```python
from build123d import *

# Parameters (mm, degrees)
SKETCH1_R               = 11
BOSS_EXTRUDE1_DEPTH     = 40
BOSS_EXTRUDE2_DEPTH     = 32
SKETCH4_W               = 144
SKETCH4_H               = 40
BOSS_EXTRUDE4_DEPTH     = 5
BOSS_EXTRUDE5_DEPTH     = 32
CUT_EXTRUDE2_DEPTH      = 3
SKETCH6_W               = 120
SKETCH6_H               = 20
CUT_EXTRUDE3_DEPTH      = 5
SKETCH8_W               = 2
SKETCH8_H               = 40
CUT_EXTRUDE_THIN1_DEPTH = 18
FILLET2_R               = 5
SKETCH9_R               = 2.25
CUT_EXTRUDE4_DEPTH      = 226
CUT_EXTRUDE5_START      = -3
CUT_EXTRUDE5_DEPTH      = 11
BOSS_EXTRUDE6_DEPTH     = 40
FILLET3_R               = 2


with BuildPart() as part:
    # Sketch1 → Boss-Extrude1 (new body)
    with BuildSketch(Plane(origin=(0, 0, 0), x_dir=(1, 0, 0), z_dir=(0, 1, 0))):
        with BuildLine():
            Line((137.460581558, -14.5), (119.460581558, -14.5))
            Line((119.460581558, -14.5), (119.460581558, 7.5))
            Line((119.460581558, 7.5), (-24.539418442, 7.5))
            Line((-24.539418442, 7.5), (-24.539418442, -14.5))
            Line((-24.539418442, -14.5), (-42.539418442, -14.5))
            Line((-42.539418442, -14.5), (-56.539418442, -14.5))
            Line((-56.539418442, -14.5), (-56.539418442, -0.5))
            ThreePointArc((-56.539418442, -0.5), (-52.438913379, 9.399494937), (-42.539418442, 13.5))
            Line((-42.539418442, 13.5), (137.460581558, 13.5))
            ThreePointArc((137.460581558, 13.5), (147.360076494, 9.399494937), (151.460581558, -0.5))
            Line((151.460581558, -0.5), (151.460581558, -14.5))
            Line((151.460581558, -14.5), (137.460581558, -14.5))
        make_face()
        with Locations((-42.539418442, -0.5)):
            Circle(SKETCH1_R, mode=Mode.SUBTRACT)
        with Locations((137.460581558, -0.5)):
            Circle(SKETCH1_R, mode=Mode.SUBTRACT)
    extrude(amount=BOSS_EXTRUDE1_DEPTH)

    # Sketch2 → Boss-Extrude2 (add)
    with BuildSketch(Plane.ZY.offset(56.539418442)):
        with BuildLine():
            Line((14.5, 40), (19, 40))
            ThreePointArc((19, 40), (22.535533906, 38.535533906), (24, 35))
            Line((24, 35), (24, 29))
            ThreePointArc((24, 29), (15, 20), (24, 11))
            Line((24, 11), (24, 5))
            ThreePointArc((24, 5), (22.535533906, 1.464466094), (19, 0))
            Line((19, 0), (14.5, 0))
            Line((14.5, 0), (14.5, 40))
        make_face()
    extrude(amount=-BOSS_EXTRUDE2_DEPTH)

    # Sketch4 → Boss-Extrude4 (add)
    with BuildSketch(Plane.XY.offset(-7.5)):
        with Locations((47.460581558, 20)):
            Rectangle(SKETCH4_W, SKETCH4_H)
    extrude(amount=BOSS_EXTRUDE4_DEPTH)

    # Sketch3 → Boss-Extrude5 (add)
    with BuildSketch(Plane(origin=(151.460581558, 0, 0), x_dir=(0, 0, -1), z_dir=(1, 0, 0))):
        with BuildLine():
            Line((-24, 11), (-24, 5))
            ThreePointArc((-24, 5), (-22.535533906, 1.464466094), (-19, 0))
            Line((-19, 0), (-14.5, 0))
            Line((-14.5, 0), (-14.5, 40))
            Line((-14.5, 40), (-19, 40))
            ThreePointArc((-19, 40), (-22.535533906, 38.535533906), (-24, 35))
            Line((-24, 35), (-24, 29))
            ThreePointArc((-24, 29), (-15, 20), (-24, 11))
        make_face()
    extrude(amount=-BOSS_EXTRUDE5_DEPTH)

    # Sketch5 → Cut-Extrude2 (cut)
    with BuildSketch(Plane(origin=(0, 0, -13.5), x_dir=(-1, 0, 0), z_dir=(0, 0, -1))):
        with BuildLine():
            Line((32.539418442, 35), (-127.460581558, 35))
            ThreePointArc((-127.460581558, 35), (-130.996115464, 33.535533906), (-132.460581558, 30))
            Line((-132.460581558, 30), (-132.460581558, 10))
            ThreePointArc((-132.460581558, 10), (-130.996115464, 6.464466094), (-127.460581558, 5))
            Line((-127.460581558, 5), (32.539418442, 5))
            ThreePointArc((32.539418442, 5), (36.074952348, 6.464466094), (37.539418442, 10))
            Line((37.539418442, 10), (37.539418442, 30))
            ThreePointArc((37.539418442, 30), (36.074952348, 33.535533906), (32.539418442, 35))
        make_face()
    extrude(amount=-CUT_EXTRUDE2_DEPTH, mode=Mode.SUBTRACT)

    # Sketch6 → Cut-Extrude3 (cut)
    with BuildSketch(Plane(origin=(0, 0, -10.5), x_dir=(-1, 0, 0), z_dir=(0, 0, -1))):
        with Locations((-47.460581558, 20)):
            Rectangle(SKETCH6_W, SKETCH6_H)
    extrude(amount=-CUT_EXTRUDE3_DEPTH, mode=Mode.SUBTRACT)

    # Sketch8 → Cut-Extrude-Thin1 (cut)
    with BuildSketch(Plane(origin=(0, 0, -13.5), x_dir=(-1, 0, 0), z_dir=(0, 0, -1))):
        with Locations((-137.460581558, 20)):
            Rectangle(SKETCH8_W, SKETCH8_H)
        with Locations((42.539418442, 20)):
            Rectangle(SKETCH8_W, SKETCH8_H)
    extrude(amount=-CUT_EXTRUDE_THIN1_DEPTH, mode=Mode.SUBTRACT)

    # Fillet2
    fillet2_edges = [part.edges().sort_by_distance(p)[0] for p in [
        (138.460581558, 0, -11.959345597),
        (138.460581558, 40, -11.959345597),
        (136.460581558, 0, -11.977225575),
        (136.460581558, 40, -11.977225575),
        (-41.539418442, 40, -11.977225575),
        (-43.539418442, 40, -11.959345597),
        (-43.539418442, 0, -11.959345597),
        (-41.539418442, 0, -11.977225575),
    ]]
    fillet(fillet2_edges, radius=FILLET2_R)

    # Sketch9 → Cut-Extrude4 (cut)
    with BuildSketch(Plane(origin=(151.460581558, 0, 0), x_dir=(0, 0, -1), z_dir=(1, 0, 0))):
        with Locations((-0.5, 20)):
            Circle(SKETCH9_R)
    extrude(amount=-CUT_EXTRUDE4_DEPTH, mode=Mode.SUBTRACT)

    # Sketch10 → Cut-Extrude5 (cut)
    with BuildSketch(Plane(origin=(-24.539418442, 0, 0), x_dir=(0, 0, -1), z_dir=(1, 0, 0)).offset(CUT_EXTRUDE5_START)):
        Polygon((-0.5, 24.156921938), (-4.1, 22.078460969), (-4.1, 17.921539031), (-0.5, 15.843078062), (3.1, 17.921539031), (3.1, 22.078460969), align=None)
    cut_extrude5 = extrude(amount=CUT_EXTRUDE5_DEPTH, mode=Mode.SUBTRACT)

    # Mirror5: Cut-Extrude5 across plane
    add(cut_extrude5.mirror(Plane.ZY.offset(-47.460581558)), mode=Mode.SUBTRACT)

    # Sketch12 → Boss-Extrude6 (add)
    with BuildSketch(Plane(origin=(0, 0, 0), x_dir=(-1, 0, 0), z_dir=(0, -1, 0))):
        with BuildLine():
            Line((-103.460581558, -3.5), (-103.460581558, 2.5))
            Line((-103.460581558, 2.5), (-100.460581558, 2.5))
            Line((-100.460581558, 2.5), (-100.460581558, -3.5))
            ThreePointArc((-100.460581558, -3.5), (-103.243067136, -10.217514421), (-109.960581558, -13))
            Line((-109.960581558, -13), (-119.460581558, -13))
            Line((-119.460581558, -13), (-119.460581558, -10))
            Line((-119.460581558, -10), (-116.460581558, -10))
            Line((-116.460581558, -10), (-109.960581558, -10))
            ThreePointArc((-109.960581558, -10), (-105.36438748, -8.096194078), (-103.460581558, -3.5))
        make_face()
    extrude(amount=-BOSS_EXTRUDE6_DEPTH)

    # Fillet3
    fillet3_edges = [part.edges().sort_by_distance(p)[0] for p in [
        (119.460581558, 20, 10),
    ]]
    fillet(fillet3_edges, radius=FILLET3_R)


solid = part.part
```
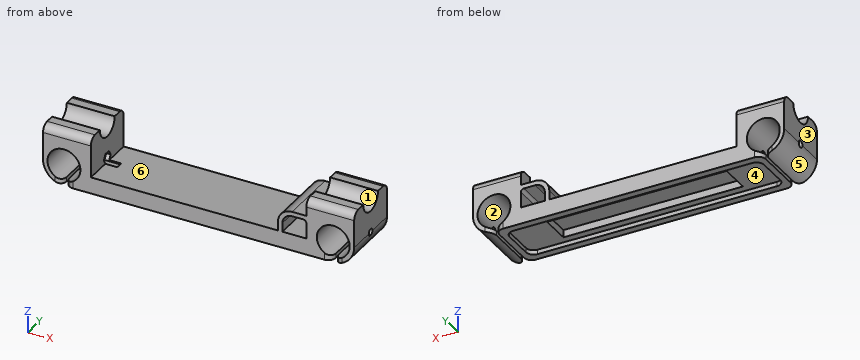
CAD build for the part. Positions are in the model's coordinates, mm. Face numbers are marked on the shaded views. A direction names the side the tool comes from. Round coordinates to 2 decimals unless told otherwise and drop trailing zeros. Loops run counter-clockwise (first coordinate to the right, second up) from the corner with the lowest first, then second, coordinate; pieces in that order, holes last. Notation, with made-up numbers: M 38,-32 L 60,-32 A18 ccw 60,-11 Z; hole C 28.5,81 d3. An arc over 180 degrees is marked long. Return JSON: item names as keys, results as strings. Group by question number.
(1) Drop flat-ended pins along their axis: P1, Ø15, axis at x = 60.5, y = 24, coming from the -Z side; P2, Ø3.5, axis at y = 20, z = 0.5, coming from the +X side; P3, Ø2.5, axis at y = 19.5, z = -11.5, coming from the -X side. Give the stop position or say it passes through.
(2) Saw through at D-D, the plane x = -21. List the corners of the cut face in (y, z), and give its area (3 significant figures).
(3) Tool access for the marked faces 4, 5 and 6: list every direction of +Z, -Z, +X, -X, +Y, -Y with a clear straight run to the whole face (end or side of a thin tool).
(4) Saw through at A-A, the plane x = 88.5. List the corners of the cut face in (y, z).
(5) Wall check: probe 1 along X at (y, z) = (29, 0); probe 2 along X at (y, z) = (5.5, -3); probe 3 along X at (y, z) = (7, 15.5). Give the ranges that are in metal, low to high. Write a range as [from, to].
(6) Mould opens along X. For the marked faces 1, 2 and 3 say: +X half, -X half, draft (parallel to the pull), parting line (faces both ways), or undercut.
(7) Saw through at B-B, the plane z = 17. List the corners of the cut face in (x, y), and give its area (3 significant figures).
Answer list:
{
 "1": {"P1": "z = -10.5", "P2": "x = 103.46", "P3": "x = -51.51"},
 "2": {"outline": "M 0,-13.5 L 5,-13.5 L 5,-10.5 L 35,-10.5 L 35,-13.5 L 40,-13.5 L 40,-2.5 L 22.42,-2.5 L 22.08,-3.1 L 17.92,-3.1 L 17.58,-2.5 L 0,-2.5 Z", "area": "347 mm2"},
 "3": {"face 4": "-Z", "face 5": "-Z, -X, +Y, -Y", "face 6": "+Z, +Y, -Y"},
 "4": {"outline": "M 0,-13.5 L 5,-13.5 L 5,-10.5 L 10,-10.5 L 10,-5.5 L 30,-5.5 L 30,-10.5 L 35,-10.5 L 35,-13.5 L 40,-13.5 L 40,-2.5 L 0,-2.5 Z"},
 "5": {"probe 1": "[-56.53, -53.53], [-31.55, -24.54], [100.46, 103.46], [119.46, 126.47], [148.45, 151.45]", "probe 2": "[-56.09, -52.97], [-32.11, 127.03], [147.89, 151.02]", "probe 3": "[-56.54, -24.54], [119.46, 151.46]"},
 "6": {"face 1": "draft", "face 2": "undercut", "face 3": "-X half"},
 "7": {"outline": "M -56.54,0 L -24.54,0 L -24.54,14.34 L -56.54,14.34 Z; M -56.54,25.66 L -24.54,25.66 L -24.54,40 L -56.54,40 Z; M 119.46,0 L 151.46,0 L 151.46,14.34 L 119.46,14.34 Z; M 119.46,25.66 L 151.46,25.66 L 151.46,40 L 119.46,40 Z", "area": "1,840 mm2"}
}
